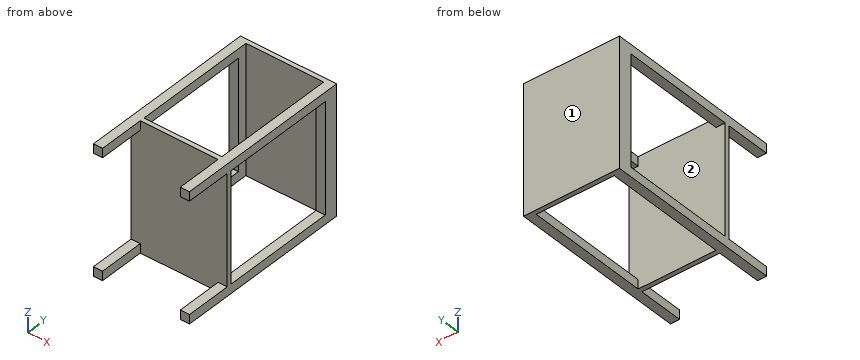
from build123d import *

# Parameters (mm, degrees)
SKETCH1_W           = 210
SKETCH1_H           = 280
BOSS_EXTRUDE1_DEPTH = 390
SKETCH4_W           = 240
SKETCH4_H           = 100
SKETCH4_H_2         = 250
CUT_EXTRUDE1_DEPTH  = 300
SKETCH5_W           = 170
SKETCH5_H           = 100
SKETCH5_H_2         = 270
CUT_EXTRUDE2_DEPTH  = 300


with BuildPart() as part:
    # Sketch1 → Boss-Extrude1 (new body)
    with BuildSketch(Plane(origin=(0, 0, 0), x_dir=(1, 0, 0), z_dir=(0, 1, 0))):
        Rectangle(SKETCH1_W, SKETCH1_H)
    extrude(amount=BOSS_EXTRUDE1_DEPTH)

    # Sketch4 → Cut-Extrude1 (cut)
    with BuildSketch(Plane(origin=(105, 0, 0), x_dir=(0, 0, -1), z_dir=(1, 0, 0))):
        with Locations((0, 50)):
            Rectangle(SKETCH4_W, SKETCH4_H)
        with Locations((0, 235)):
            Rectangle(SKETCH4_W, SKETCH4_H_2)
    extrude(amount=-CUT_EXTRUDE1_DEPTH, mode=Mode.SUBTRACT)

    # Sketch5 → Cut-Extrude2 (cut)
    with BuildSketch(Plane.XY.offset(140)):
        with Locations((0, 50)):
            Rectangle(SKETCH5_W, SKETCH5_H)
        with Locations((0, 245)):
            Rectangle(SKETCH5_W, SKETCH5_H_2)
    extrude(amount=-CUT_EXTRUDE2_DEPTH, mode=Mode.SUBTRACT)


solid = part.part
Verification items for the finished model (mm, model axes). Face numbers are marked on the shaded views. Round coordinates to 2 decimals unless told otherwise and drop trailing zeros. Loops run counter-clockwise (first coordinate to the right, second up) from the corner with the lowest first, then second, coordinate; pieces in that order, holes last. Notation, with made-up numbers: (17, 19) - (38, 19) arc R9 cw to (38, 24) - close; hole circle Ø10 at (73.25, 3). An arc over 180 degrees is marked (long way). Use a Markdown table: item, result. Add a question column.
1. Section check A-A, the plane z = -29.5. Record the boundary of the cut face in (x, y), plus the area to 3 significant figures.
2. Thickness scan on probe 1 along X at (y, z) = (241, -126.5); probe 2 along Y at (x, z) = (-32.5, 37); probe 3 along Z at (x, y) = (-96, 132). Record the ranges inside material, lowest first. Write a range as [from, to].
3. Section check D-D, the plane y = 241.5. Record the boundary of the cut face in (x, z).
4. Section check C-C, the plane y = 366. Record the boundary of the cut face in (x, z), plus the area to 3 significant figures.
5. Section check B-B, the plane x = -40.5. Record the boundary of the cut face in (y, z).
6. Release check for a two-part mould opening along Z. For the marked faces 1 and 2 record: released by +Z, released by -Z, zero draft, split by the parting line, or undercut.
7. Gauge pin test, flat end, axial feed: pin 1 (4 mm diameter, centred on x = -38.5, z = -9.5, fed in from -Y). Record the tip position at first contact, or that the pin passes through.
Checks:
| question | item | result |
|---|---|---|
| 1 | outline | (-105, 100) - (105, 100) - (105, 110) - (-105, 110) - close; (-105, 360) - (-85, 360) - (-85, 380) - (85, 380) - (85, 360) - (105, 360) - (105, 390) - (-105, 390) - close |
| 1 | area | 5,000 mm^2 |
| 2 | probe 1 | x = [-105, -85], [85, 105] |
| 2 | probe 2 | y = [100, 110], [380, 390] |
| 2 | probe 3 | z = [-140, -120], [120, 140] |
| 3 | outline | (-105, -140) - (-85, -140) - (-85, -120) - (-105, -120) - close; (-105, 120) - (-85, 120) - (-85, 140) - (-105, 140) - close; (85, -140) - (105, -140) - (105, -120) - (85, -120) - close; (85, 120) - (105, 120) - (105, 140) - (85, 140) - close |
| 4 | outline | (-105, -140) - (-85, -140) - (-85, 140) - (-105, 140) - close; (85, -140) - (105, -140) - (105, 140) - (85, 140) - close |
| 4 | area | 11,200 mm^2 |
| 5 | outline | (100, -140) - (110, -140) - (110, 140) - (100, 140) - close; (380, -140) - (390, -140) - (390, 140) - (380, 140) - close |
| 6 | face 1 | zero draft |
| 6 | face 2 | undercut |
| 7 | pin 1 | stops at y = 100 |
